Read the model definition and answer for the solid it produces. Units are mm, in the model's axes. Round coordinates to 2 decimals unless told otherwise and drop trailing zeros. Loops run counter-clockwise (first coordinate to the right, second up) from the corner with the lowest first, then second, coordinate; pieces in that order, holes last. Notation, with made-up numbers: (10.25, 33) - (54.25, 33) arc R29 cw to (54.25, 59) - close; hole circle Ø3 at (26.5, 49). An arc over 180 degrees is marked (long way). Answer as CSV lines item,"result".
Autodesk Inventor part; units mm, degrees
ref_plane "YZ Plane" through (0, 0, 0) normal (1, 0, 0) x (0, 1, 0)
ref_plane "XZ Plane" through (0, 0, 0) normal (0, 1, 0) x (-1, 0, 0)
ref_plane "XY Plane" through (0, 0, 0) normal (0, 0, 1) x (1, 0, 0)
sketch "Sketch1" plane through (0, 0, 0) normal (0, 0, 1) x (1, 0, 0)
  line L0 (-34.036, -29.7688) -> (34.036, -29.7688)
  line L1 (34.036, -29.7688) -> (34.036, 29.7688)
  line L2 (34.036, 29.7688) -> (-34.036, 29.7688)
  line L3 (-34.036, 29.7688) -> (-34.036, -29.7688)
  line L4 (-34.036, -29.7688) -> (34.036, 29.7688) construction
  line L5 (34.036, -29.7688) -> (-34.036, 29.7688) construction
  point P0 (0, 0)
  dimension "d0" = 68.072
  dimension "d1" = 59.5376
extrude "Extrusion1" add sketch "Sketch1" along normal blind 6.35
sketch "Sketch3" plane through (0, 0, 6.35) normal (0, 0, 1) x (1, 0, 0)
  line L0 (34.036, 29.7688) -> (-34.036, 29.7688)
  line L1 (-34.036, -29.7688) -> (34.036, -29.7688)
  line L2 (-34.036, 29.7688) -> (-34.036, -29.7688)
  line L3 (34.036, -29.7688) -> (34.036, 29.7688)
  point P0 (0, 0)
  point P1 (-18.796, 8.1788)
  point P2 (-18.796, -8.1788)
  point P3 (18.796, -8.1788)
  point P4 (18.796, 8.1788)
  point P5 (0, 8.1788)
  point P6 (0, -8.1788)
  dimension "d17" = 21.59
  dimension "d18" = 21.59
  dimension "d19" = 15.24
  dimension "d20" = 15.24
  dimension "d21" = 18.796
  dimension "d23" = 37.592
hole "Hole2" at (-18.796, 8.1788, 6.35) at (-18.796, -8.1788, 6.35) at (18.796, -8.1788, 6.35) at (18.796, 8.1788, 6.35) at (0, 8.1788, 6.35) at (0, -8.1788, 6.35) direction (0, 0, -1) diameter 3 depth 25.4 tip angle 118 countersink diameter 5.6 countersink angle 90
chamfer "Chamfer1" distance 8.89 angle 45 2 edges at (-34.036, -29.7688, 3.175) (34.036, -29.7688, 3.175)
sketch "Sketch4" plane through (0, 0, 0) normal (0, 0, -1) x (-1, 0, 0)
  circle A0 centre (-14.605, -25.4024) radius 1.7018
  circle A1 centre (14.605, -25.4024) radius 1.7018
  circle A2 centre (14.605, 25.3976) radius 1.7018
  circle A3 centre (-14.605, 25.3976) radius 1.7018
  point P0 (0, 0)
hole "Hole3" at (14.605, -25.4024, 0) at (-14.605, -25.4024, 0) at (-14.605, 25.3976, 0) at (14.605, 25.3976, 0) direction (0, 0, 1) diameter 3.4036 end through all countersink diameter 6.2992 countersink angle 90
properties part number "DPLX_P032_VIPE Insulation Middle" material "Polyethylene, High Density"
1) Find the intervals of material crossed by line 1 (Y direction, x = 14.5, z = 6.25); line 2 (X direction, y = 26, z = 1); line 3 (X direction, y = -26.5, z = 0.75), in increasing order.
Entries:
line 1,"y = -29.77 to -27.1, -23.7 to 23.7, 27.1 to 29.77"
line 2,"x = -34.04 to -16.67, -12.54 to 12.54, 16.67 to 34.04"
line 3,"x = -28.41 to -16.74, -12.47 to 12.47, 16.74 to 28.41"
2) The mould has two halves that part along Y. Classify faces 1 (the face through (0.575, -9.564, 2.49)), 2 (the face through (0, 29.769, 3)), 3 (the face through (-34.036, 5, 3)): pulls with the +Y half, pulls with the -Y half, needs draft (parallel to the pull), parting line crosses it, or undercut.
Entries:
face 1,"undercut"
face 2,"pulls with the +Y half"
face 3,"needs draft"
3) A cutting plane is placed at A-A, the plane x = 0. Determine the outline of the cut face in (y, z).
Entries:
outline,"(-29.77, 0) - (-9.68, 0) - (-9.68, 5.05) - (-10.98, 6.35) - (-29.77, 6.35) - close; (-6.68, 0) - (6.68, 0) - (6.68, 5.05) - (5.38, 6.35) - (-5.38, 6.35) - (-6.68, 5.05) - close; (9.68, 0) - (29.77, 0) - (29.77, 6.35) - (10.98, 6.35) - (9.68, 5.05) - close"
4) A cutting plane is placed at B-B, the plane z = 4.25. Count the separate pieces of the cut face and the enclosed holes in it, plus the area to 4 significant figures.
Entries:
separate pieces,"1"
enclosed holes,"10"
area,"3,895 mm^2"
5) Each of these flat-tipped pins is pushed along its axis until it touches: P1, Ø1.8, axis at x = 18.8, y = 8.18, coming from the +Z side; P2, Ø3.5, axis at x = 18.8, y = -8.18, coming from the -Z side; P3, Ø5.5, axis at x = -14.6, y = -25.4, coming from the -Z side; P4, Ø4.5, axis at x = 14.6, y = -25.4, coming from the -Z side. Where does it stop, or does it pass through?
Entries:
P1,"passes through"
P2,"stops at z = 0"
P3,"stops at z = 0.39"
P4,"stops at z = 0.89"
